```python
from build123d import *
from build123d.topology import SkipClean

# Parameters (mm, degrees)
BOSS_EXTRUDE1_DEPTH     = 4
SKETCH2_W               = 19.302325582
SKETCH2_H               = 17
BOSS_EXTRUDE2_DEPTH     = 3
CUT_EXTRUDE1_DEPTH      = 52.89534967
CUT_EXTRUDE1_DEPTH_BACK = 52.89534967
BOSS_EXTRUDE3_DEPTH     = 17
FILLET1_R               = 3
CUT_EXTRUDE2_DEPTH      = 50.194156235
CUT_EXTRUDE2_DEPTH_BACK = 50.194156235
SKETCH5_R               = 1.5
CUT_EXTRUDE3_DEPTH      = 52.662994567
CUT_EXTRUDE3_DEPTH_BACK = 52.662994567
SKETCH6_R               = 1.5
FILLET2_R               = 3
SKETCH7_R               = 2.75
CUT_EXTRUDE5_DEPTH      = 50.194156235


with BuildPart() as part:
    # Sketch1 → Boss-Extrude1 (new body)
    with BuildSketch(Plane.XY):
        Polygon((-28.357138738, -40), (-18.357138738, -40), (9.651162791, 0), (-9.651162791, 0), align=None)
    extrude(amount=BOSS_EXTRUDE1_DEPTH)

    # Sketch2 → Boss-Extrude2 (add)
    with BuildSketch(Plane(origin=(0, 0, 0), x_dir=(1, 0, 0), z_dir=(0, 1, 0))):
        with Locations((0, -2)):
            Rectangle(SKETCH2_W, SKETCH2_H)
    extrude(amount=BOSS_EXTRUDE2_DEPTH)

    # Sketch3 → Cut-Extrude1 (cut, two sides: drawn at the far end of the back side and taken through both)
    with BuildSketch(Plane.XY.offset(10.5).offset(-CUT_EXTRUDE1_DEPTH_BACK)):
        Polygon((-9.651162791, 0), (-8.248214595, 3), (-9.651162791, 3), align=None)
    extrude(amount=CUT_EXTRUDE1_DEPTH + CUT_EXTRUDE1_DEPTH_BACK, mode=Mode.SUBTRACT)

    # Sketch4 → Boss-Extrude3 (add, through all)
    with BuildSketch(Plane.XY.offset(10.5)):
        Polygon((9.651162791, 3), (9.651162791, 0), (11.751785405, 3), align=None)
    extrude(amount=-BOSS_EXTRUDE3_DEPTH)

    # Fillet1
    fillet1_edges = [part.edges().sort_by_distance(p)[0] for p in [
        (-18.357138738, -40, 2),
        (-28.357138738, -40, 2),
    ]]
    fillet(fillet1_edges, radius=FILLET1_R)

    # Sketch5 → Cut-Extrude2 (cut, two sides: drawn at the far end of the back side and taken through both)
    with BuildSketch(Plane.XY.offset(4).offset(-CUT_EXTRUDE2_DEPTH_BACK)):
        with Locations((-17.517854053, -30)):
            Circle(SKETCH5_R)
        Polygon((-10.732268808, -23.880216821), (-17.506894929, -23.880216821), (-2.185708769, -11.674464137), align=None)
        Polygon((-14.648109244, -17.767120785), (3.88821641, -3), (-7.742274088, -3), align=None)
    extrude(amount=CUT_EXTRUDE2_DEPTH + CUT_EXTRUDE2_DEPTH_BACK, mode=Mode.SUBTRACT)

    # Sketch6 → Cut-Extrude3 (cut, two sides: drawn at the far end of the back side and taken through both)
    with BuildSketch(Plane(origin=(0, 3, 0), x_dir=(1, 0, 0), z_dir=(0, 1, 0)).offset(-CUT_EXTRUDE3_DEPTH_BACK)):
        with Locations(Location((-4.248214595, 2.75, 0), (0, 0, 180))):
            Circle(SKETCH6_R)
        with Locations(Location((7.751785405, -6.75, 0), (0, 0, 180))):
            Circle(SKETCH6_R)
    extrude(amount=CUT_EXTRUDE3_DEPTH + CUT_EXTRUDE3_DEPTH_BACK, mode=Mode.SUBTRACT)

    # Fillet2
    # the kernel refuses this fillet: 3 mm, written as the material it adds along each edge
    with BuildSketch(Plane(origin=(17.151162791, 0, 0), x_dir=(0, -1, 0), z_dir=(-1, 0, 0))) as fillet2_piece_1_section:
        with BuildLine():
            CenterArc((FILLET2_R, -FILLET2_R), FILLET2_R, 90, 90)
            Line((0, -FILLET2_R), (0, 0))
            Line((0, 0), (FILLET2_R, 0))
        make_face()
    fillet2_piece_1 = extrude(amount=34.302325581, mode=Mode.PRIVATE)
    fillet2_piece_1 = split(fillet2_piece_1, bisect_by=Plane(origin=(8.707650451, -1.347475267, -0.62141613), z_dir=(-0.8191520442889888, 0.5735764363510504, 0)), keep=Keep.TOP, mode=Mode.PRIVATE)
    fillet2_piece_1 = split(fillet2_piece_1, bisect_by=Plane(origin=(-6.80101607, 6.094622871, -0.62141613), z_dir=(0.9058417102512069, -0.42361633109356, 0)), keep=Keep.TOP, mode=Mode.PRIVATE)
    fillet2_piece_1 = fillet2_piece_1 - Plane(origin=(-4.248214595, -0.776972683, -2.75), x_dir=(-1, 0, 0), z_dir=(0, 1, 0)) * Cylinder(1.5, 81, mode=Mode.PRIVATE)
    add(fillet2_piece_1)
    with BuildSketch(Plane(origin=(17.151162791, 0, 4), x_dir=(0, -1, 0), z_dir=(-1, 0, 0))) as fillet2_piece_2_section:
        with BuildLine():
            CenterArc((FILLET2_R, FILLET2_R), FILLET2_R, 180, 90)
            Line((0, FILLET2_R), (0, 0))
            Line((0, 0), (FILLET2_R, 0))
        make_face()
    fillet2_piece_2 = extrude(amount=34.302325581, mode=Mode.PRIVATE)
    fillet2_piece_2 = split(fillet2_piece_2, bisect_by=Plane(origin=(8.664647852, -1.408889344, 4.489642882), z_dir=(-0.8191520442889888, 0.5735764363510504, 0)), keep=Keep.TOP, mode=Mode.PRIVATE)
    fillet2_piece_2 = split(fillet2_piece_2, bisect_by=Plane(origin=(-6.833394213, 6.025386936, 4.489642882), z_dir=(0.9058417102512069, -0.42361633109356, 0)), keep=Keep.TOP, mode=Mode.PRIVATE)
    fillet2_piece_2 = fillet2_piece_2 - Plane(origin=(7.751785405, -0.84697785, 6.75), x_dir=(-1, 0, 0), z_dir=(0, 1, 0)) * Cylinder(1.5, 81, mode=Mode.PRIVATE)
    add(fillet2_piece_2)

    # Sketch7 → Cut-Extrude5 (cut, through all)
    with SkipClean():  # the faces are left unmerged after this step: merging them gives an invalid solid
        with BuildSketch(Plane.XZ):
            with Locations((-4.248214595, -2.75)):
                Circle(SKETCH7_R)
            with Locations((7.751785405, 6.75)):
                Circle(SKETCH7_R)
        extrude(amount=CUT_EXTRUDE5_DEPTH, mode=Mode.SUBTRACT)


solid = part.part
```
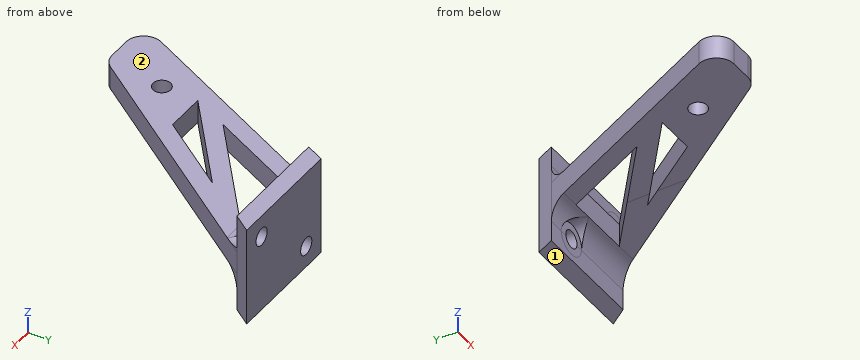
Could you check a few things on this model? Use its own coordinates, in mm. Face numbers are marked on the shaded views. A direction names the side the tool comes from. Give positions to 0.01 mm unless a question says otherwise; leave off trailing zeros. Write each loop counter-clockwise with the first axis right and the second up, starting at its lowest first coordinate (ties: lowest second). Pieces come first, ordered by that corner, then holes. Notation, with made-up numbers: (86, 7) - (125, 7) arc R32 ccw to (125, 41) - close; hole circle Ø7 at (2, -28.5). An arc over 180 degrees is marked (long way). One line per item, written item: value. Start each with the question number.
Item 1: Please list where these lines run through material, in increasing order: line 1 (Y direction, x = -4.5, z = 0.5); line 2 (Z direction, x = -9, y = -5); line 3 (Y direction, x = -6, z = 8). Write a range as from..to.
Item 2: Imagine slicing it at A-A, the plane x = -9. List the corners of the cut face in (y, z) for me, and give its area (3 significant figures).
Item 3: I'm going to push flat-ended pins straight in: pin 1 (8 mm diameter, centred on x = -19, y = -15.5, fed in from -Z); pin 2 (1.1 mm diameter, centred on x = -1.5, z = -5, fed in from -Y); pin 3 (0.9 mm diameter, centred on x = 8, z = 6, fed in from -Y); pin 4 (2.5 mm diameter, centred on x = -4, z = -1, fed in from -Y). Where does each tip first touch, or does it pass through?
Item 4: Which directions (+Z, -Z, +X, -X, +Y, -Y) give clear straight access to the entire face, cutting with the end or side of a thin tool? Please do the marked faces 1 and 2.
Item 5: Imagine slicing it at D-D, the plane x = 0.5. List the corners of the cut face in (y, z) for me, and give its area (3 significant figures).
Item 6: Imagine slicing it at B-B, the plane y = -30. List the corners of the cut face in (x, z) for me, and give its area (3 significant figures).
Item 7: Imagine slicing it at C-C, the plane z = 2. List the corners of the cut face in (x, y) for me, and give its area (3 significant figures).
Geometry says:
1. line 1: -20.21..-14.98, -13.52..-9.68, -3..3
1. line 2: 0..4
1. line 3: 0..3
2. outline: (-26.64, 0) - (-21.41, 0) - (-21.41, 4) - (-26.64, 4) - close; (-17.1, 0) - (-13.27, 0) - (-13.27, 4) - (-17.1, 4) - close; (-5.69, 0) - (-3, 0) arc R3 cw to (0, -3) - (0, -6.5) - (1.39, -6.5) - (1.39, 10.5) - (0, 10.5) - (0, 7) arc R3 cw to (-3, 4) - (-5.69, 4) - close
2. area: 86.6 mm^2
3. pin 1: z = 0
3. pin 2: y = 0
3. pin 3: through
3. pin 4: y = -20.57
4. face 1: -Z, +X, -X, +Y, -Y
4. face 2: +Z, +X, -X, -Y
5. outline: (-13.07, 0) - (-5.7, 0) - (-5.7, 4) - (-13.07, 4) - close; (-3, 0) arc R3 cw to (0, -3) - (0, -6.5) - (3, -6.5) - (3, 10.5) - (0, 10.5) - (0, 7) arc R3 cw to (-3, 4) - close
5. area: 96.3 mm^2
6. outline: (-23.68, 0) - (-19.02, 0) - (-19.02, 4) - (-23.68, 4) - close; (-16.02, 0) - (-11.36, 0) - (-11.36, 4) - (-16.02, 4) - close
6. area: 37.3 mm^2
7. outline: (-26.36, -35.73) arc R3 ccw to (-23.64, -40) - (-19.92, -40) arc R3 ccw to (-17.46, -38.72) - (11.75, 3) - (-8.25, 3) - close; hole circle Ø3 at (-17.52, -30); hole (-17.51, -23.88) - (-10.73, -23.88) - (-2.19, -11.67) - close; hole (-14.65, -17.77) - (3.89, -3) - (-7.74, -3) - close
7. area: 505 mm^2
